Geometry check sheet. Reference: the model listing, model coordinates, mm. Round coordinates to 2 decimals unless told otherwise and drop trailing zeros. Order: outer loops, then holes, each group sorted by start corner. A loop starts at its lowest first (then second) coordinate and runs counter-clockwise, first axis right, second up. Notation, with made-up numbers: (36.25, -25.75) -> (44.25, -25.75) arc R5 cw to (44.25, -19.75) -> close; hole circle Ø6 at (82, 15.25). An arc over 180 degrees is marked (long way). Answer as a JSON object with one key per item and string values. Group by question number.
from build123d import *

# Parameters (mm, degrees)
BOSS_EXTRUDE1_DEPTH   = 1.5
F_4_0MM_DOWEL_HOLE1_D = 3.3
SKETCH4_W             = 12.7
SKETCH4_H             = 6.35
CUT_EXTRUDE1_DEPTH    = 1.5
FILLET1_R             = 2


with BuildPart() as part:
    # Sketch1 → Boss-Extrude1 (new body)
    with BuildSketch(Plane(origin=(0, 0, 0), x_dir=(1, 0, 0), z_dir=(0, 1, 0))):
        Polygon((0, 0), (104.14, 0), (104.140084457, -68.379681711), (114.300084457, -68.379681711), (114.300084457, -97.679681711), (104.140084457, -97.679681711), (104.140084457, -126.999681711), (52.560084457, -126.999681711), (0, -67.34), align=None)
    extrude(amount=BOSS_EXTRUDE1_DEPTH)

    # Ø4.0mm Dowel Hole1 (through all)
    with Locations(Plane(origin=(5.08, 1.5, 5.08), x_dir=(0, 0, 1), z_dir=(0, 1, 0))):
        with Locations((0, 0), (0, 47.95), (0, 93.980006274), (116.839681711, 93.980084457), (116.839681711, 50.770084457), (89.156056724, 25.385630403), (58, 0)):
            Hole(F_4_0MM_DOWEL_HOLE1_D / 2)

    # Sketch4 → Cut-Extrude1 (cut)
    with BuildSketch(Plane(origin=(0, 1.5, 0), x_dir=(1, 0, 0), z_dir=(0, 1, 0))):
        with Locations((69, -13.335)):
            Rectangle(SKETCH4_W, SKETCH4_H)
    extrude(amount=-CUT_EXTRUDE1_DEPTH, mode=Mode.SUBTRACT)

    # Fillet1
    fillet1_edges = [part.edges().sort_by_distance(p)[0] for p in [
        (62.65, 0.75, 10.16),
        (62.65, 0.75, 16.51),
        (75.35, 0.75, 16.51),
        (75.35, 0.75, 10.16),
    ]]
    fillet(fillet1_edges, radius=FILLET1_R)


solid = part.part
Item 1: Sectioned sample at D-D, the plane x = 5.08. Enter the section's corners in (y, z), then the cut area to 3 significant figures.
Item 2: Sectioned sample at C-C, the plane y = 0.6. Count the separate pieces of the cut face and the enclosed holes in it, then the cut area to 3 significant figures.
Item 3: Depth check by flat-ended pin: pin 1 Ø0.8 at (y, z) = (1, 13) entering from -X. Enter the tip coordinate at first touch or a pass-through.
Item 4: Sectioned sample at B-B, the plane z = 5.08. Enter the section's corners in (x, y), then the cut area to 3 significant figures.
Item 5: Mould release check, pull along Z, two halves, no side actions. Record for faces 1 (the flat face through (26.65, 0.74, 97.59)), 2 (the flat face through (58, 0, 63)), 3 (the cylindrical face through (97.45, 0.74, 5.44)): pulls with the +Z half, pulls with the -Z half, needs draft (parallel to the pull), parting line crosses it, or undercut.
Item 6: Thickness scan on L1, parallel to X at y = 1.15, z = 5.08; L2, parallel to X at y = 0.85, z = 63.08; L3, parallel to X at y = 0.6, z = 95. Record the ranges inside material, lowest first.
Item 7: Sectioned sample at A-A, the plane z = 63.08. Enter the section's corners in (x, y), then the cut area to 3 significant figures.
Result:
{
 "1": {"outline": "(0, 0) -> (1.5, 0) -> (1.5, 3.43) -> (0, 3.43) -> close; (0, 6.73) -> (1.5, 6.73) -> (1.5, 61.43) -> (0, 61.43) -> close; (0, 64.73) -> (1.5, 64.73) -> (1.5, 73.11) -> (0, 73.11) -> close", "area": "99.8 mm2"},
 "2": {"separate pieces": "1", "enclosed holes": "8", "area": "11,800 mm2"},
 "3": {"pin 1": "stops at x = 0"},
 "4": {"outline": "(0, 0) -> (3.43, 0) -> (3.43, 1.5) -> (0, 1.5) -> close; (6.73, 0) -> (51.38, 0) -> (51.38, 1.5) -> (6.73, 1.5) -> close; (54.68, 0) -> (97.41, 0) -> (97.41, 1.5) -> (54.68, 1.5) -> close; (100.71, 0) -> (104.14, 0) -> (104.14, 1.5) -> (100.71, 1.5) -> close", "area": "141 mm2"},
 "5": {"face 1": "pulls with the +Z half", "face 2": "needs draft", "face 3": "undercut"},
 "6": {"L1": "x = 0 to 3.43, 6.73 to 51.38, 54.68 to 97.41, 100.71 to 104.14", "L2": "x = 0 to 3.43, 6.73 to 104.14", "L3": "x = 24.37 to 29, 31.93 to 114.3"},
 "7": {"outline": "(0, 0) -> (3.43, 0) -> (3.43, 1.5) -> (0, 1.5) -> close; (6.73, 0) -> (104.14, 0) -> (104.14, 1.5) -> (6.73, 1.5) -> close", "area": "151 mm2"}
}
